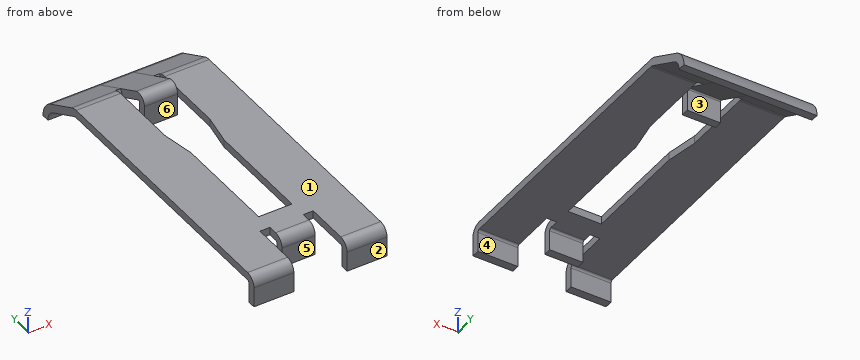
from build123d import *

# Parameters (mm, degrees)
MAIN_PLATE_DEPTH               = 0.35
EDGE_FLANGE1_STRIP_W           = 1.6
EDGE_FLANGE1_STRIP_H           = 0.35
EDGE_FLANGE1_STRIP_CUT_DEPTH   = 1.8
EDGE_FLANGE1_STRIP_2_W         = 1.6
EDGE_FLANGE1_STRIP_2_H         = 0.35
EDGE_FLANGE1_STRIP_CUT_2_DEPTH = 1.8
EDGE_FLANGE1_STRIP_3_W         = 1.6
EDGE_FLANGE1_STRIP_3_H         = 0.35
EDGE_FLANGE1_STRIP_CUT_3_DEPTH = 1.5
EDGE_FLANGE1_DEPTH             = 1.8
EDGE_FLANGE1_BEND_DEPTH        = 1.8
EDGE_FLANGE1_BEND_2_DEPTH      = 1.5
CENTRAL_SECTION_DEPTH          = 0.75
BOSS_EXTRUDE3_DEPTH            = 2.25
BOSS_EXTRUDE4_START            = -2.25
BOSS_EXTRUDE4_DEPTH            = 2.25
SKETCH20_W                     = 0.25
SKETCH20_H                     = 0.4
CUT_EXTRUDE1_DEPTH             = 1


# Sheet-metal steps are written as plain solids
with BuildPart() as part:
    # Sketch1 → Main Plate (new body)
    with BuildSketch(Plane.XY):
        Polygon((-3, 9.4), (-3, -2.85), (-1.2, -2.85), (-1.2, -0.8), (-0.75, -0.8), (-0.75, -1.3), (0.75, -1.3), (0.75, -0.8), (1.2, -0.8), (1.2, -2.85), (3, -2.85), (3, 9.4), (1, 9.4), (1, 6.217820455), (0.75, 4.8), (0.75, 0), (-0.75, 0), (-0.75, 4.8), (-1, 6.217820455), (-1, 9.4), align=None)
    extrude(amount=-MAIN_PLATE_DEPTH)

    # Edge-Flange1 strip (across the edge) → Edge-Flange1 strip cut (cut)
    with BuildSketch(Plane(origin=(3, -2.85, -0.35), x_dir=(0, 1, 0), z_dir=(-1, 0, 0))):
        with Locations((-0.7, -0.175)):
            Rectangle(EDGE_FLANGE1_STRIP_W, EDGE_FLANGE1_STRIP_H)
    extrude(amount=EDGE_FLANGE1_STRIP_CUT_DEPTH, mode=Mode.SUBTRACT)

    # Edge-Flange1 strip 2 (across the edge) → Edge-Flange1 strip cut 2 (cut)
    with BuildSketch(Plane(origin=(-1.2, -2.85, -0.35), x_dir=(0, 1, 0), z_dir=(-1, 0, 0))):
        with Locations((-0.7, -0.175)):
            Rectangle(EDGE_FLANGE1_STRIP_2_W, EDGE_FLANGE1_STRIP_2_H)
    extrude(amount=EDGE_FLANGE1_STRIP_CUT_2_DEPTH, mode=Mode.SUBTRACT)

    # Edge-Flange1 strip 3 (across the edge) → Edge-Flange1 strip cut 3 (cut)
    with BuildSketch(Plane(origin=(0.75, -1.3, -0.35), x_dir=(0, 1, 0), z_dir=(-1, 0, 0))):
        with Locations((-0.7, -0.175)):
            Rectangle(EDGE_FLANGE1_STRIP_3_W, EDGE_FLANGE1_STRIP_3_H)
    extrude(amount=EDGE_FLANGE1_STRIP_CUT_3_DEPTH, mode=Mode.SUBTRACT)

    # Edge-Flange1 section (across the edge) → Edge-Flange1 (add)
    with BuildSketch(Plane(origin=(3, -2.85, -0.35), x_dir=(0, 1, 0), z_dir=(-1, 0, 0))):
        with BuildLine():
            Line((-0.35, 0.1), (-0.35, 1))
            Line((-0.35, 1), (0, 1))
            Line((0, 1), (0, 0.1))
            ThreePointArc((0, 0.1), (0.029289322, 0.029289322), (0.1, 0))
            Line((0.1, 0), (0.1, -0.35))
            ThreePointArc((0.1, -0.35), (-0.218198052, -0.218198052), (-0.35, 0.1))
        make_face()
    extrude(amount=EDGE_FLANGE1_DEPTH)

    # Edge-Flange1 section 2 (across the edge) → Edge-Flange1 bend (add)
    with BuildSketch(Plane(origin=(-1.2, -2.85, -0.35), x_dir=(0, 1, 0), z_dir=(-1, 0, 0))):
        with BuildLine():
            Line((-0.35, 0.1), (-0.35, 1))
            Line((-0.35, 1), (0, 1))
            Line((0, 1), (0, 0.1))
            ThreePointArc((0, 0.1), (0.029289322, 0.029289322), (0.1, 0))
            Line((0.1, 0), (0.1, -0.35))
            ThreePointArc((0.1, -0.35), (-0.218198052, -0.218198052), (-0.35, 0.1))
        make_face()
    extrude(amount=EDGE_FLANGE1_BEND_DEPTH)

    # Edge-Flange1 section 3 (across the edge) → Edge-Flange1 bend 2 (add)
    with BuildSketch(Plane(origin=(0.75, -1.3, -0.35), x_dir=(0, 1, 0), z_dir=(-1, 0, 0))):
        with BuildLine():
            Line((-0.35, 0.1), (-0.35, 1))
            Line((-0.35, 1), (0, 1))
            Line((0, 1), (0, 0.1))
            ThreePointArc((0, 0.1), (0.029289322, 0.029289322), (0.1, 0))
            Line((0.1, 0), (0.1, -0.35))
            ThreePointArc((0.1, -0.35), (-0.218198052, -0.218198052), (-0.35, 0.1))
        make_face()
    extrude(amount=EDGE_FLANGE1_BEND_2_DEPTH)



with BuildPart() as body_2:
    # Sketch15 → Central Section (new, symmetric)
    with BuildSketch(Plane(origin=(0, 0, 0), x_dir=(0, 0, -1), z_dir=(1, 0, 0))):
        with BuildLine():
            Line((0.9, 8.1), (0.9, 8.45))
            Line((0.9, 8.45), (-0.1, 8.45))
            ThreePointArc((-0.1, 8.45), (-0.14270772, 8.473999025), (-0.144417693, 8.522957973))
            Line((-0.144417693, 8.522957973), (1.160923854, 11.048453645))
            ThreePointArc((1.160923854, 11.048453645), (1.400341198, 11.305200355), (1.738353869, 11.4))
            Line((1.738353869, 11.4), (1.738353869, 11.75))
            ThreePointArc((1.738353869, 11.75), (1.218334376, 11.604154393), (0.85, 11.209159454))
            Line((0.85, 11.209159454), (-0.455341547, 8.683663782))
            ThreePointArc((-0.455341547, 8.683663782), (-0.441661757, 8.291992203), (-0.1, 8.1))
            Line((-0.1, 8.1), (0.9, 8.1))
        make_face()
    extrude(amount=CENTRAL_SECTION_DEPTH, both=True)


with BuildPart() as part_1:
    add(part.part)

    add(body_2.part)  # Boss-Extrude3 merges body 2
    # Sketch16 → Boss-Extrude3 (add)
    with BuildSketch(Plane(origin=(3, 0, 0), x_dir=(0, 0, -1), z_dir=(1, 0, 0))):
        with BuildLine():
            Line((0.35, 9.4), (0, 9.4))
            ThreePointArc((0, 9.4), (0.019169334, 9.55996991), (0.075591878, 9.710881579))
            Line((0.075591878, 9.710881579), (0.85, 11.209159454))
            ThreePointArc((0.85, 11.209159454), (1.218334376, 11.604154393), (1.738353869, 11.75))
            Line((1.738353869, 11.75), (1.738353869, 11.4))
            ThreePointArc((1.738353869, 11.4), (1.400341198, 11.305200355), (1.160923854, 11.048453645))
            Line((1.160923854, 11.048453645), (0.386515732, 9.55017577))
            ThreePointArc((0.386515732, 9.55017577), (0.359260019, 9.477275741), (0.35, 9.4))
        make_face()
    extrude(amount=-BOSS_EXTRUDE3_DEPTH)

    # Sketch19 → Boss-Extrude4 (add)
    with BuildSketch(Plane.ZY.offset(3).offset(BOSS_EXTRUDE4_START)):
        with BuildLine():
            Line((-0.35, 9.4), (0, 9.4))
            ThreePointArc((0, 9.4), (-0.019169334, 9.55996991), (-0.075591878, 9.710881579))
            Line((-0.075591878, 9.710881579), (-0.85, 11.209159454))
            ThreePointArc((-0.85, 11.209159454), (-1.218334376, 11.604154393), (-1.738353869, 11.75))
            Line((-1.738353869, 11.75), (-1.738353869, 11.4))
            ThreePointArc((-1.738353869, 11.4), (-1.400341198, 11.305200355), (-1.160923854, 11.048453645))
            Line((-1.160923854, 11.048453645), (-0.386515732, 9.55017577))
            ThreePointArc((-0.386515732, 9.55017577), (-0.359260019, 9.477275741), (-0.35, 9.4))
        make_face()
    extrude(amount=BOSS_EXTRUDE4_DEPTH)

    # Sketch20 → Cut-Extrude1 (cut)
    with BuildSketch(Plane(origin=(0, 2.016486324, 3.901375463), x_dir=(1, 0, 0), z_dir=(0, 0.4591594538479162, 0.8883538686481212))):
        with Locations((0.875, 8.550526365)):
            Rectangle(SKETCH20_W, SKETCH20_H)
        with Locations((-0.875, 8.550526365)):
            Rectangle(SKETCH20_W, SKETCH20_H)
    extrude(amount=-CUT_EXTRUDE1_DEPTH, mode=Mode.SUBTRACT)


solid = part_1.part
CAD build for the part. Positions are in the model's coordinates, mm. Face numbers are marked on the shaded views. A direction names the side the tool comes from. Give positions to 0.01 mm unless a question says otherwise; leave off trailing zeros. Write each loop counter-clockwise with the first axis right and the second up, starting at its lowest first coordinate (ties: lowest second). Pieces come first, ordered by that corner, then holes. Notation, with made-up numbers: (27.5, -38) - (43.5, -38) arc R27 cw to (43.5, -17) - close; hole circle Ø10 at (65, 41.5). An arc over 180 degrees is marked (long way). Put each result on its own line as item: value.
(1) Saw through at A-A (y = 3). List the corners of the cut face in (x, z), then the cut area to 4 significant figures.
Working result:
outline: (-3, -0.35) - (-0.75, -0.35) - (-0.75, 0) - (-3, 0) - close; (0.75, -0.35) - (3, -0.35) - (3, 0) - (0.75, 0) - close
area: 1.575 mm^2
(2) Tool access for the marked faces 4, 5 and 6: list every direction of +Z, -Z, +X, -X, +Y, -Y with a clear straight run to the whole face (end or side of a thin tool).
Working result:
face 4: -Z, +X, -X
face 5: +Z, -Z, +X, -X, -Y
face 6: +Z, -Z
(3) Saw through at C-C (y = 8.25). List the corners of the cut face in (x, z).
Working result:
outline: (-3, -0.35) - (-1, -0.35) - (-1, 0) - (-3, 0) - close; (-0.75, -0.9) - (0.75, -0.9) - (0.75, 0.41) - (-0.75, 0.41) - close; (1, -0.35) - (3, -0.35) - (3, 0) - (1, 0) - close
(4) Pull direction Y, two halves, no side cores. Call the marked faces 1, 2 and 3: released by +Y, released by -Y, zero draft, split by the parting line, or undercut.
Working result:
face 1: zero draft
face 2: released by -Y
face 3: undercut
(5) Saw through at D-D (x = 2.45). List the corners of the cut face in (y, z).
Working result:
outline: (-3.2, -1.35) - (-2.85, -1.35) - (-2.85, -0.45) arc R0.1 cw to (-2.75, -0.35) - (9.4, -0.35) arc R0.33 cw to (9.55, -0.39) - (11.05, -1.16) arc R0.65 cw to (11.4, -1.74) - (11.75, -1.74) arc R1 ccw to (11.21, -0.85) - (9.71, -0.08) arc R0.68 ccw to (9.4, 0) - (-2.75, 0) arc R0.45 ccw to (-3.2, -0.45) - close
(6) Drop flat-ended pins along their axis: pin 1 Ø1 at (y, z) = (2, -1) entering from +X; pin 2 Ø0.7 at (y, z) = (-1, -1) entering from +X; pin 3 Ø0.7 at (x, z) = (0, -1) entering from +Y; pin 4 Ø1.5 at (x, y) = (2, 8) entering from -Z. Give the stop position or say it passes through.
Working result:
pin 1: through
pin 2: x = 0.75
pin 3: y = 11.67
pin 4: z = -0.35
(7) Wall check: L1, parallel to X at y = -2.5, z = -0.2; L2, parallel to Z at x = -2.5, y = -0.5. Give the ranges that are in metal, low to high.
Working result:
L1: -3 to -1.2, 1.2 to 3
L2: -0.35 to 0
(8) Saw through at B-B (x = 0.2). List the corners of the cut face in (y, z).
Working result:
outline: (-1.65, -1.35) - (-1.3, -1.35) - (-1.3, -0.45) arc R0.1 cw to (-1.2, -0.35) - (0, -0.35) - (0, 0) - (-1.2, 0) arc R0.45 ccw to (-1.65, -0.45) - close; (8.1, -0.9) - (8.45, -0.9) - (8.45, 0.1) arc R0.05 cw to (8.52, 0.14) - (11.05, -1.16) arc R0.65 cw to (11.4, -1.74) - (11.75, -1.74) arc R1 ccw to (11.21, -0.85) - (8.68, 0.46) arc R0.4 ccw to (8.1, 0.1) - close
